Work out the finished part from the listing and answer in its coordinate system (mm). Round coordinates to 2 decimals unless told otherwise and drop trailing zeros. Loops run counter-clockwise (first coordinate to the right, second up) from the corner with the lowest first, then second, coordinate; pieces in that order, holes last. Notation, with made-up numbers: (73.5, 5) - (115.5, 5) arc R14 ccw to (115.5, 30) - close; hole circle Ø2 at (-29, -27). An arc over 180 degrees is marked (long way). Answer as CSV lines item,"result". Start each with the question number.
Q1. Section C-C on y = 4 is taken. Count the separate pieces of the cut face and the enclosed holes in it, then the cut area to 3 significant figures.
Q2. Straight lines are drawn through the part: L1, parallel to Z at x = 40.5, y = 2; L2, parallel to Z at x = 14, y = 3.25; L3, parallel to Z at x = 6, y = 6.75. For each, find the intervals that lie inside material, in ascending order. Write a range as [from, to].
Q3. Section B-B on z = 10.5 is taken. Write down the section's boundary in (x, y).
Q4. Each of these flat-tipped pins is pushed along its axis until it touches: pin 1 Ø1.6 at (x, z) = (45.96, 14.47) entering from -Y; pin 2 Ø2.5 at (y, z) = (2, -180.5) entering from +X; pin 3 Ø1.5 at (x, y) = (-26.5, 5.5) entering from -Z; pin 4 Ø1.5 at (x, z) = (31, 18.5) entering from +Y. Where does it stop, or does it pass through?
Q5. Section A-A on z = -203 is taken. Write down the section's boundary in (x, y).
```python
from build123d import *

# Parameters (mm, degrees)
SKETCH1_R                 = 8.89
BOSS_EXTRUDE1_DEPTH       = 8.382
FILLET3_R                 = 1.27
TAP_DRILL_FOR_6_32_TAP2_D = 2.7051
LPATTERN1_COUNT           = 2
LPATTERN1_PITCH           = 44.39
LPATTERN1_COUNT_DIR2      = 2
LPATTERN1_PITCH_DIR2      = 64.59
TAP_DRILL_FOR_6_32_TAP3_D = 2.7051
TAP_DRILL_FOR_6_32_TAP5_D = 2.7051
CUT_EXTRUDE2_DEPTH        = 231.337524251
CUT_EXTRUDE2_DEPTH_BACK   = 2.54


with BuildPart() as part:
    # Sketch1 → Boss-Extrude1 (new body)
    with BuildSketch(Plane(origin=(0, 0, 0), x_dir=(1, 0, 0), z_dir=(0, 1, 0))):
        with BuildLine():
            Line((-15.926997076, 220.899744797), (43.763002924, 220.899744797))
            ThreePointArc((43.763002924, 220.899744797), (46.457079761, 219.783821634), (47.573002924, 217.089744797))
            Line((47.573002924, 217.089744797), (47.573002924, 190.419744797))
            ThreePointArc((47.573002924, 190.419744797), (46.457079761, 187.725667961), (43.763002924, 186.609744797))
            Line((43.763002924, 186.609744797), (39.953002924, 186.609744797))
            ThreePointArc((39.953002924, 186.609744797), (37.258926088, 185.493821634), (36.143002924, 182.799744797))
            Line((36.143002924, 182.799744797), (36.143002924, 177.719744797))
            ThreePointArc((36.143002924, 177.719744797), (37.258926088, 175.025667961), (39.953002924, 173.909744797))
            Line((39.953002924, 173.909744797), (60.908002924, 173.909744797))
            ThreePointArc((60.908002924, 173.909744797), (63.602079761, 172.793821634), (64.718002924, 170.099744797))
            Line((64.718002924, 170.099744797), (64.718002924, -51.515255203))
            Line((64.718002924, -51.515255203), (52.272002924, -51.515255203))
            Line((52.272002924, -51.515255203), (49.413478553, -59.368986367))
            ThreePointArc((49.413478553, -59.368986367), (48.483543444, -60.580901395), (47.026659296, -61.040255203))
            Line((47.026659296, -61.040255203), (-19.190653447, -61.040255203))
            ThreePointArc((-19.190653447, -61.040255203), (-20.647537596, -60.580901395), (-21.577472704, -59.368986367))
            Line((-21.577472704, -59.368986367), (-24.435997076, -51.515255203))
            Line((-24.435997076, -51.515255203), (-36.881997076, -51.515255203))
            Line((-36.881997076, -51.515255203), (-36.881997076, 170.099744797))
            ThreePointArc((-36.881997076, 170.099744797), (-35.766073912, 172.793821634), (-33.071997076, 173.909744797))
            Line((-33.071997076, 173.909744797), (-12.116997076, 173.909744797))
            ThreePointArc((-12.116997076, 173.909744797), (-9.422920239, 175.025667961), (-8.306997076, 177.719744797))
            Line((-8.306997076, 177.719744797), (-8.306997076, 182.799744797))
            ThreePointArc((-8.306997076, 182.799744797), (-9.422920239, 185.493821634), (-12.116997076, 186.609744797))
            Line((-12.116997076, 186.609744797), (-15.926997076, 186.609744797))
            ThreePointArc((-15.926997076, 186.609744797), (-18.621073912, 187.725667961), (-19.736997076, 190.419744797))
            Line((-19.736997076, 190.419744797), (-19.736997076, 217.089744797))
            ThreePointArc((-19.736997076, 217.089744797), (-18.621073912, 219.783821634), (-15.926997076, 220.899744797))
        make_face()
        with Locations(Location((13.918002924, 203.754744797, 0), (0, 0, 270))):
            Circle(SKETCH1_R, mode=Mode.SUBTRACT)
    extrude(amount=BOSS_EXTRUDE1_DEPTH)

    # Fillet3
    fillet3_edges = [part.edges().sort_by_distance(p)[0] for p in [
        (-36.881997076, 4.191, 51.515255203),
        (64.718002924, 4.191, 51.515255203),
    ]]
    fillet(fillet3_edges, radius=FILLET3_R)

    # Tap Drill for #6-32 Tap2 (through all)
    with Locations(Plane(origin=(0, 8.382, 0), x_dir=(1, 0, 0), z_dir=(0, 1, 0))):
        with Locations((-18.626997076, -14.470255203)):
            tap_drill_for_6_32_tap2 = Hole(TAP_DRILL_FOR_6_32_TAP2_D / 2)

    # LPattern1: Tap Drill for _6-32 Tap2 2 × 2
    with Locations(*[(j * LPATTERN1_PITCH_DIR2, 0, -i * LPATTERN1_PITCH) for i in range(LPATTERN1_COUNT) for j in range(LPATTERN1_COUNT_DIR2) if (i, j) != (0, 0)]):
        add(tap_drill_for_6_32_tap2, mode=Mode.SUBTRACT)

    # Tap Drill for #6-32 Tap3 (through all)
    with Locations(Plane(origin=(0, 8.382, 0), x_dir=(1, 0, 0), z_dir=(0, 1, 0))):
        with Locations((-31.251997076, 11.924744797), (59.088002924, 11.924744797)):
            Hole(TAP_DRILL_FOR_6_32_TAP3_D / 2)

    # Tap Drill for #6-32 Tap5 (through all)
    with Locations(Plane(origin=(0, 8.382, 0), x_dir=(1, 0, 0), z_dir=(0, 1, 0))):
        with Locations((-32.451997076, -28.700255203), (60.288002924, -28.700255203)):
            Hole(TAP_DRILL_FOR_6_32_TAP5_D / 2)

    # Sketch2 → Cut-Extrude2 (cut, two sides: drawn at the far end of the back side and taken through both)
    with BuildSketch(Plane(origin=(0, 8.382, 0), x_dir=(1, 0, 0), z_dir=(0, 1, 0)).offset(-CUT_EXTRUDE2_DEPTH_BACK)):
        with BuildLine():
            Line((-0.076281623, -26.570255203), (0.413729291, -26.570255203))
            Line((0.413729291, -26.570255203), (0.413729291, -5.470255203))
            Line((0.413729291, -5.470255203), (-2.245226951, -5.470255203))
            ThreePointArc((-2.245226951, -5.470255203), (-4.485024518, -16.361968965), (-0.076281623, -26.570255203))
        make_face()
        Polygon((3.413729291, -26.570255203), (13.918002924, -26.570255203), (24.266068116, -26.570255203), (24.266068116, -5.470255203), (13.918002924, -5.470255203), (3.413729291, -5.470255203), align=None)
        with BuildLine():
            Line((27.266068116, -5.470255203), (27.266068116, -26.570255203))
            Line((27.266068116, -26.570255203), (27.912287472, -26.570255203))
            ThreePointArc((27.912287472, -26.570255203), (31.255019163, -20.926095035), (32.418002924, -14.470255203))
            ThreePointArc((32.418002924, -14.470255203), (31.824283285, -9.821048426), (30.081232799, -5.470255203))
            Line((30.081232799, -5.470255203), (27.266068116, -5.470255203))
        make_face()
    extrude(amount=CUT_EXTRUDE2_DEPTH + CUT_EXTRUDE2_DEPTH_BACK, mode=Mode.SUBTRACT)


solid = part.part
```
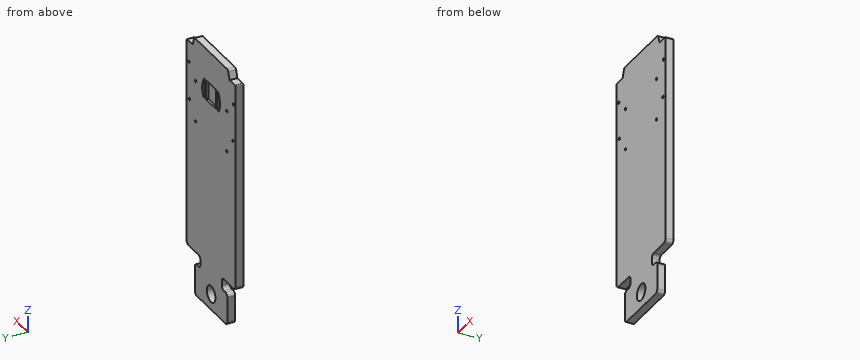
Findings:
1,separate pieces,"1"
1,enclosed holes,"9"
1,area,"26,200 mm^2"
2,L1,"z = [-220.9, -186.61], [-173.91, 61.04]"
2,L2,"z = [-220.9, -212.64], [-194.87, 61.04]"
2,L3,"z = [-220.9, -207.8], [-199.71, 5.47], [26.57, 61.04]"
3,outline,"(-36.88, 0) - (64.72, 0) - (64.72, 8.38) - (31.99, 8.38) - (31.99, 5.84) - (27.27, 5.84) - (27.27, 8.38) - (24.27, 8.38) - (24.27, 5.84) - (3.41, 5.84) - (3.41, 8.38) - (0.41, 8.38) - (0.41, 5.84) - (-4.15, 5.84) - (-4.15, 8.38) - (-36.88, 8.38) - close"
4,pin 1,"passes through"
4,pin 2,"stops at x = 36.14"
4,pin 3,"stops at z = -173.91"
4,pin 4,"stops at y = 5.84"
5,outline,"(-19.74, 0) - (5.06, 0) - (5.06, 8.38) - (-19.74, 8.38) - close; (22.78, 0) - (47.57, 0) - (47.57, 8.38) - (22.78, 8.38) - close"
